```python
from build123d import *

# Parameters (mm, degrees)
F0_R     = 15
F0_R_2   = 1.5
F1_DEPTH = 3
F2_R     = 15
F2_R_2   = 10
F3_DEPTH = 4


with BuildPart() as f1:
    # F0 (on Top) → F1 (new body)
    with BuildSketch(Plane.XY):
        Circle(F0_R)
        with Locations((0, -7.5)):
            Circle(F0_R_2, mode=Mode.SUBTRACT)
        with Locations((-7.5, 0)):
            Circle(F0_R_2, mode=Mode.SUBTRACT)
        with BuildLine():
            ThreePointArc((4, 0), (-2.8284271247, -2.8284271247), (0, 4))
            ThreePointArc((0, 4), (2.8284271247, 2.8284271247), (4, 0))
        make_face(mode=Mode.SUBTRACT)
        with Locations((7.5, 0)):
            Circle(F0_R_2, mode=Mode.SUBTRACT)
        with BuildLine():
            ThreePointArc((1.5, 7.5), (1.0606601718, 6.4393398282), (0, 6))
            ThreePointArc((0, 6), (-1.0606601718, 8.5606601718), (1.5, 7.5))
        make_face(mode=Mode.SUBTRACT)
    extrude(amount=F1_DEPTH)

    # F2 (on face) → F3 (join)
    with BuildSketch(Plane.XY.offset(3)):
        Circle(F2_R)
        Circle(F2_R_2, mode=Mode.SUBTRACT)
    extrude(amount=F3_DEPTH)


solid = f1.part
```
Geometry check sheet. Reference: the model listing, model coordinates, mm. A direction names the side the tool comes from. Coordinates: 2 decimals unless noted, no trailing zeros. Loops run counter-clockwise (first coordinate to the right, second up) from the corner with the lowest first, then second, coordinate; pieces in that order, holes last.
Item 1: Sectioned sample at D-D, the plane y = 11.75. Record the boundary of the cut face in (x, z), then the cut area to 3 significant figures.
Item 2: Sectioned sample at C-C, the plane z = 4. Record the boundary of the cut face in (x, y).
Item 3: Sectioned sample at B-B, the plane y = -7.5. Record the boundary of the cut face in (x, z).
Item 4: Thickness scan on line 1 (Y direction, x = 0, z = 2.1); line 2 (Z direction, x = -5, y = 2.25); line 3 (X direction, y = 2, z = 6.75). Record the ranges inside material, lowest first.
Item 5: Access from +Z, -Z, +X, -X, +Y, -Y to the whole of each face (thin tool, end or side, straight path). Record for faces 4 (the face through (0, -9, 1)), 5 (the face through (-2.17, -9.76, 4.97)).
Item 6: Go/stop test with flat-tipped pins: pin 1 Ø4 at (y, z) = (6.5, 3) entering from -X; pin 2 Ø9 at (x, y) = (0, 0) entering from +Z; pin 3 Ø2.5 at (x, y) = (0, -7.5) entering from +Z; pin 4 Ø1 at (y, z) = (-5.5, 1.5) entering from -X. Record where each tip stops, or that it passes through.
Item 7: Sectioned sample at A-A, the plane x = -6.5. Record the boundary of the cut face in (y, z).
Item 8: Release check for a two-part mould opening along Y. For faces 1 (the face through (-14.985, 0.66, 3.451)), 2 (the face through (3, -10, 7)), 3 (the face through (-9, 0, 1)) record: released by +Y, released by -Y, zero draft, split by the parting line, or undercut.
Check result:
1. outline: (-9.32, 0) - (9.32, 0) - (9.32, 7) - (-9.32, 7) - close
1. area: 131 mm2
2. outline: circle Ø30 at (0, 0); hole circle Ø20 at (0, 0)
3. outline: (-12.99, 0) - (-1.5, 0) - (-1.5, 3) - (-6.61, 3) - (-6.61, 7) - (-12.99, 7) - close; (1.5, 0) - (12.99, 0) - (12.99, 7) - (6.61, 7) - (6.61, 3) - (1.5, 3) - close
4. line 1: y = -15 to -9, -6 to -4, 4 to 6, 9 to 15
4. line 2: z = 0 to 3
4. line 3: x = -14.87 to -9.8, 9.8 to 14.87
5. face 4: +Z, -Z
5. face 5: +Z
6. pin 1: stops at x = -14.31
6. pin 2: stops at z = 3
6. pin 3: passes through
6. pin 4: stops at x = -14.14
7. outline: (-13.52, 0) - (-1.12, 0) - (-1.12, 3) - (-7.6, 3) - (-7.6, 7) - (-13.52, 7) - close; (1.12, 0) - (13.52, 0) - (13.52, 7) - (7.6, 7) - (7.6, 3) - (1.12, 3) - close
8. face 1: split by the parting line
8. face 2: zero draft
8. face 3: undercut
